For this review, take the finished solid that the model builds, in its own axes (mm). Face numbers are marked on the shaded views. A direction names the side the tool comes from. Give positions to 0.01 mm unless a question says otherwise; leave off trailing zeros. Loops run counter-clockwise (first coordinate to the right, second up) from the corner with the lowest first, then second, coordinate; pieces in that order, holes last. Notation, with made-up numbers: (23, -35.5) -> (80, -35.5) arc R7 ccw to (80, -28.5) -> close; hole circle Ø5 at (50, -23.75). An arc over 180 degrees is marked (long way). One line per question, with ' | ' between items. Start each with the question number.
(1) Consider section C-C (z = -31.5). Write out the cut boundary in (x, y), and give its area (3 significant figures).
(2) Draft analysis for pull direction Z (two halves, no side actions). For the marked faces 3, 4 and 5, state which applies: +Z half, -Z half, draft (parallel to the pull), parting line (faces both ways), or undercut.
(3) Tool access review of the marked faces 1 and 2: name each direction out of +Z, -Z, +X, -X, +Y, -Y from which nothing blocks a thin tool from reaching the whole face with its end or side.
(4) Consider section D-D (x = -134). Write out the cut boundary in (y, z).
(5) Wall thickness on probe 1 along X at (y, z) = (75.8, -43); probe 2 along Z at (x, y) = (-153, 85); probe 3 along Y at (x, z) = (-151, -51.5): over which ranges is each line inside the solid? List them lowest first.
(6) Insertion check: P1, Ø1, axis at x = -148.5, z = -24.5, coming from the +Y side; P2, Ø2.5, axis at x = -150.41, y = 75.8, coming from the -Z side; P3, Ø3.5, axis at x = -122.41, y = 116, coming from the -Z side. Each pin has a flat end and moves straight along its axis. Give the tip position at first contact, or say it passes through.
(7) Consider section B-B (y = 116). Write out the cut boundary in (x, z), and give its area (3 significant figures).
(8) Consider section A-A (y = 88). Write out the cut boundary in (x, z), and give its area (3 significant figures).
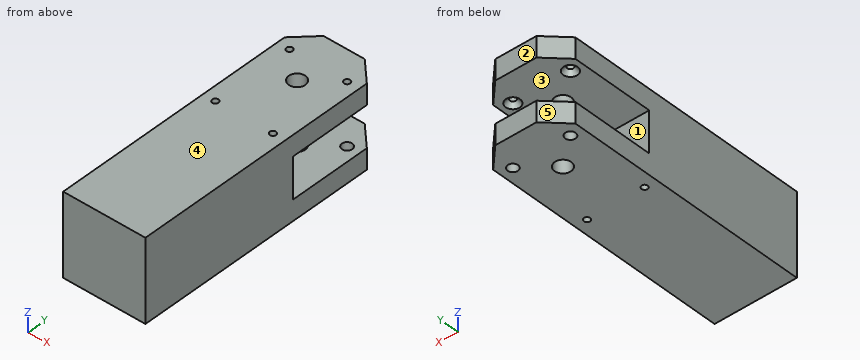
from build123d import *

# Parameters (mm, degrees)
SKETCH1_W           = 40
SKETCH1_H           = 40
BOSS_EXTRUDE1_DEPTH = 80
SKETCH4_W           = 40
SKETCH4_H           = 10
BOSS_EXTRUDE2_DEPTH = 50
CHAMFER1_SIZE       = 10
SKETCH5_R           = 4
CUT_EXTRUDE1_DEPTH  = 60
SKETCH6_R           = 1.5
CUT_EXTRUDE2_DEPTH  = 60
CHAMFER2_SIZE       = 2
SKETCH7_R           = 2.5
CUT_EXTRUDE3_DEPTH  = 20


with BuildPart() as part:
    # Sketch1 → Boss-Extrude1 (new body)
    with BuildSketch(Plane(origin=(0, 0, 0), x_dir=(1, 0, 0), z_dir=(0, 1, 0))):
        with Locations((-136.41025641, 40.096153846)):
            Rectangle(SKETCH1_W, SKETCH1_H)
    extrude(amount=BOSS_EXTRUDE1_DEPTH)

    # Sketch4 → Boss-Extrude2 (add)
    with BuildSketch(Plane(origin=(0, 80, 0), x_dir=(1, 0, 0), z_dir=(0, 1, 0))):
        with Locations((-136.41025641, 25.096153846)):
            Rectangle(SKETCH4_W, SKETCH4_H)
        with Locations((-136.41025641, 55.096153846)):
            Rectangle(SKETCH4_W, SKETCH4_H)
    extrude(amount=BOSS_EXTRUDE2_DEPTH)

    # Chamfer1
    chamfer1_edges = [part.edges().sort_by_distance(p)[0] for p in [
        (-156.41025641, 130, -25.096153846),
        (-116.41025641, 130, -25.096153846),
        (-156.41025641, 130, -55.096153846),
        (-116.41025641, 130, -55.096153846),
    ]]
    chamfer(chamfer1_edges, length=CHAMFER1_SIZE)

    # Sketch5 → Cut-Extrude1 (cut)
    with BuildSketch(Plane(origin=(0, 0, -60.096153846), x_dir=(-1, 0, 0), z_dir=(0, 0, -1))):
        with Locations((136.41025641, 104.479752215)):
            Circle(SKETCH5_R)
    extrude(amount=-CUT_EXTRUDE1_DEPTH, mode=Mode.SUBTRACT)

    # Sketch6 → Cut-Extrude2 (cut)
    with BuildSketch(Plane.XY.offset(-20.096153846)):
        with Locations((-150.41025641, 75.8)):
            Circle(SKETCH6_R)
        with Locations((-150.41025641, 116)):
            Circle(SKETCH6_R)
        with Locations((-122.41025641, 116)):
            Circle(SKETCH6_R)
        with Locations((-122.41025641, 75.8)):
            Circle(SKETCH6_R)
    extrude(amount=-CUT_EXTRUDE2_DEPTH, mode=Mode.SUBTRACT)

    # Chamfer2
    chamfer2_edges = [part.edges().sort_by_distance(p)[0] for p in [
        (-123.91025641, 116, -30.096153846),
        (-151.91025641, 116, -30.096153846),
    ]]
    chamfer(chamfer2_edges, length=CHAMFER2_SIZE)

    # Sketch7 → Cut-Extrude3 (cut)
    with BuildSketch(Plane(origin=(0, 0, -60.096153846), x_dir=(-1, 0, 0), z_dir=(0, 0, -1))):
        with Locations((150.41025641, 116)):
            Circle(SKETCH7_R)
        with Locations((122.41025641, 116)):
            Circle(SKETCH7_R)
    extrude(amount=-CUT_EXTRUDE3_DEPTH, mode=Mode.SUBTRACT)


solid = part.part
A:
1) outline: (-156.41, 0) -> (-116.41, 0) -> (-116.41, 80) -> (-156.41, 80) -> close; hole circle Ø3 at (-150.41, 75.8); hole circle Ø3 at (-122.41, 75.8) | area: 3,190 mm^2
2) face 3: undercut | face 4: +Z half | face 5: draft
3) face 1: +X, -X, +Y | face 2: +Z, -Z, +X, -X, +Y
4) outline: (0, -60.1) -> (101.29, -60.1) -> (101.29, -50.1) -> (80, -50.1) -> (80, -30.1) -> (101.29, -30.1) -> (101.29, -20.1) -> (0, -20.1) -> close; (107.67, -60.1) -> (130, -60.1) -> (130, -50.1) -> (107.67, -50.1) -> close; (107.67, -30.1) -> (130, -30.1) -> (130, -20.1) -> (107.67, -20.1) -> close
5) probe 1: x = -156.41 to -151.91, -148.91 to -123.91, -120.91 to -116.41 | probe 2: z = -60.1 to -50.1, -30.1 to -20.1 | probe 3: y = 0 to 74.42, 77.18 to 113.57, 118.43 to 125.41
6) P1: stops at y = 128.41 | P2: passes through | P3: stops at z = -28.35
7) outline: (-156.41, -60.1) -> (-152.91, -60.1) -> (-152.91, -50.1) -> (-156.41, -50.1) -> close; (-156.41, -30.1) -> (-153.91, -30.1) -> (-151.91, -28.1) -> (-151.91, -20.1) -> (-156.41, -20.1) -> close; (-148.91, -28.1) -> (-146.91, -30.1) -> (-125.91, -30.1) -> (-123.91, -28.1) -> (-123.91, -20.1) -> (-148.91, -20.1) -> close; (-147.91, -60.1) -> (-124.91, -60.1) -> (-124.91, -50.1) -> (-147.91, -50.1) -> close; (-120.91, -28.1) -> (-118.91, -30.1) -> (-116.41, -30.1) -> (-116.41, -20.1) -> (-120.91, -20.1) -> close; (-119.91, -60.1) -> (-116.41, -60.1) -> (-116.41, -50.1) -> (-119.91, -50.1) -> close | area: 632 mm^2
8) outline: (-156.41, -60.1) -> (-116.41, -60.1) -> (-116.41, -50.1) -> (-156.41, -50.1) -> close; (-156.41, -30.1) -> (-116.41, -30.1) -> (-116.41, -20.1) -> (-156.41, -20.1) -> close | area: 800 mm^2
